The model under review builds one solid part; all positions refer to its coordinate system, in mm. A direction names the side the tool comes from. Round coordinates to 2 decimals unless told otherwise and drop trailing zeros. Loops run counter-clockwise (first coordinate to the right, second up) from the corner with the lowest first, then second, coordinate; pieces in that order, holes last. Notation, with made-up numbers: (-13.5, -30.75) -> (39.5, -30.75) arc R17 cw to (39.5, 1.25) -> close; hole circle Ø2 at (8, 55.5). An arc over 180 degrees is marked (long way). Return JSON: item names as keys, results as strings. Group by question number.
```python
from build123d import *

# Parameters (mm, degrees)
BOSS_EXTRUDE1_DEPTH = 35
SKETCH2_R           = 1.75
SKETCH2_W           = 11.6
SKETCH2_H           = 22.75
CUT_EXTRUDE1_DEPTH  = 1.59
SKETCH4_R           = 1.25
CUT_EXTRUDE3_DEPTH  = 4
SKETCH5_R           = 1
CUT_EXTRUDE4_DEPTH  = 4


with BuildPart() as part:
    # Sketch1 → Boss-Extrude1 (new body)
    with BuildSketch(Plane(origin=(0, 0, 0), x_dir=(1, 0, 0), z_dir=(0, 1, 0))):
        Polygon((0, -13), (1.59, -13), (1.59, -1.59), (16.59, -1.59), (16.59, -28.41), (1.59, -28.41), (1.59, -17), (0, -17), (0, -30), (18.18, -30), (18.18, 0), (0, 0), align=None)
    extrude(amount=BOSS_EXTRUDE1_DEPTH)

    # Sketch2 → Cut-Extrude1 (cut)
    with BuildSketch(Plane(origin=(0, 0, 0), x_dir=(-1, 0, 0), z_dir=(0, 0, -1))):
        with Locations((-9.09, 32.375)):
            Circle(SKETCH2_R)
        with Locations((-9.09, 2.625)):
            Circle(SKETCH2_R)
        with Locations((-9.09, 17.5)):
            Rectangle(SKETCH2_W, SKETCH2_H)
    extrude(amount=-CUT_EXTRUDE1_DEPTH, mode=Mode.SUBTRACT)

    # Sketch4 → Cut-Extrude3 (cut)
    with BuildSketch(Plane.ZY):
        with Locations((6.5, 11.22)):
            Circle(SKETCH4_R)
        with Locations((23.5, 11.22)):
            Circle(SKETCH4_R)
    extrude(amount=-CUT_EXTRUDE3_DEPTH, mode=Mode.SUBTRACT)

    # Sketch5 → Cut-Extrude4 (cut)
    with BuildSketch(Plane.XY.offset(30)):
        with Locations((9.09, 11.22)):
            Circle(SKETCH5_R)
    extrude(amount=-CUT_EXTRUDE4_DEPTH, mode=Mode.SUBTRACT)


solid = part.part
```
1. Wall thickness on line 1 (X direction, y = 28.5, z = 1.75); line 2 (Z direction, x = 16.5, y = 4); line 3 (Y direction, x = 9.09, z = 0.95) (3 decimals): over which ranges is each line inside the solid? List them lowest first.
2. We need section A-A, the plane x = 9.09. Write out the cut boundary in (y, z) (3 decimals), then the cut area to 3 significant figures.
3. We need section C-C, the plane z = 10. Write out the cut boundary in (x, y), then the cut area to 3 significant figures.
4. We need section D-D, the plane x = 5.75. Write out the cut boundary in (y, z) (3 decimals), then the cut area to 3 significant figures.
5. Draft analysis for pull direction Z (two halves, no side actions). For faces 6 (the face through (16.59, 17, 15)), 7 (the face through (15.3, 17.3, 0)), 8 (the face through (9, 17, 30)), state which applies: pulls with the +Z half, pulls with the -Z half, needs draft (parallel to the pull), parting line crosses it, or undercut.
6. Tool access review of faces 1 (the face through (0.78, 10, 6.23)), 2 (the face through (10.38, 33.56, 0.78)), 3 (the face through (17, 0, 15)), 4 (the face through (1.59, 17, 23)), 5 (the face through (8.09, 11.26, 29.22)): name each direction out of +Z, -Z, +X, -X, +Y, -Y from which nothing blocks a thin tool from reaching the whole face with its end or side.
7. We need section B-B, the plane y = 11.22. Write out the cut boundary in (x, z).
8. For P1, Ø2, axis at x = 15, z = 18, coming from the -Y side; P2, Ø1.5, axis at x = 9, y = 25, coming from the -Z side, all flat-tipped, find the tip position at first contact; note any pin that passes through.
Check sheet entries:
{
 "1": {"line 1": "x = 0 to 1.59, 16.59 to 18.18", "line 2": "z = 0 to 1.59, 28.41 to 30", "line 3": "y = 0 to 0.875, 4.375 to 6.125, 28.875 to 30.625, 34.125 to 35"},
 "2": {"outline": "(0, 0) -> (0.875, 0) -> (0.875, 1.59) -> (0, 1.59) -> close; (0, 28.41) -> (10.22, 28.41) -> (10.22, 30) -> (0, 30) -> close; (4.375, 0) -> (6.125, 0) -> (6.125, 1.59) -> (4.375, 1.59) -> close; (12.22, 28.41) -> (35, 28.41) -> (35, 30) -> (12.22, 30) -> close; (28.875, 0) -> (30.625, 0) -> (30.625, 1.59) -> (28.875, 1.59) -> close; (34.125, 0) -> (35, 0) -> (35, 1.59) -> (34.125, 1.59) -> close", "area": "60.8 mm²"},
 "3": {"outline": "(0, 0) -> (1.59, 0) -> (1.59, 35) -> (0, 35) -> close; (16.59, 0) -> (18.18, 0) -> (18.18, 35) -> (16.59, 35) -> close", "area": "111 mm²"},
 "4": {"outline": "(0, 0) -> (6.125, 0) -> (6.125, 1.59) -> (0, 1.59) -> close; (0, 28.41) -> (35, 28.41) -> (35, 30) -> (0, 30) -> close; (28.875, 0) -> (35, 0) -> (35, 1.59) -> (28.875, 1.59) -> close", "area": "75.1 mm²"},
 "5": {"face 6": "undercut", "face 7": "pulls with the -Z half", "face 8": "pulls with the +Z half"},
 "6": {"face 1": "-X", "face 2": "-Z", "face 3": "+Z, -Z, +X, -X, -Y", "face 4": "+Y, -Y", "face 5": "+Z, -Z"},
 "7": {"outline": "(0, 0) -> (3.29, 0) -> (3.29, 1.59) -> (1.59, 1.59) -> (1.59, 5.25) -> (0, 5.25) -> close; (0, 7.75) -> (1.59, 7.75) -> (1.59, 13) -> (0, 13) -> close; (0, 17) -> (1.59, 17) -> (1.59, 22.25) -> (0, 22.25) -> close; (0, 24.75) -> (1.59, 24.75) -> (1.59, 28.41) -> (8.09, 28.41) -> (8.09, 30) -> (0, 30) -> close; (10.09, 28.41) -> (16.59, 28.41) -> (16.59, 1.59) -> (14.89, 1.59) -> (14.89, 0) -> (18.18, 0) -> (18.18, 30) -> (10.09, 30) -> close"},
 "8": {"P1": "passes through", "P2": "stops at z = 28.41"}
}
